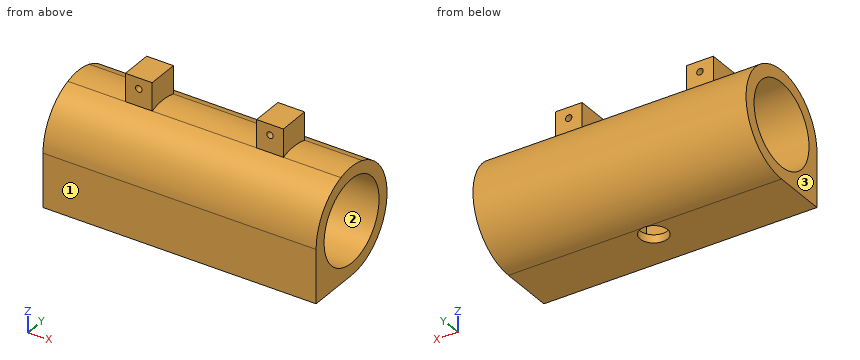
from build123d import *

# Parameters (mm, degrees)
SKETCH1_W                = 34
SKETCH1_H                = 30
BOSS_EXTRUDE2_DEPTH      = 51
SKETCH3_R                = 2.55
CUT_EXTRUDE3_DEPTH       = 10
SKETCH5_R                = 7.75
CUT_EXTRUDE4_DEPTH       = 51
SKETCH6_W                = 7
SKETCH6_H                = 30
CUT_EXTRUDE6_DEPTH       = 51
CUT_EXTRUDE7_DEPTH       = 51
CUT_EXTRUDE9_DEPTH       = 1.5
CUT_EXTRUDE9_DEPTH_BACK  = 1.5
BOSS_EXTRUDE5_DEPTH      = 51
CUT_EXTRUDE10_DEPTH      = 13
CUT_EXTRUDE11_DEPTH      = 13
SKETCH13_W               = 2
SKETCH13_H               = 6
CUT_EXTRUDE12_DEPTH      = 2
CUT_EXTRUDE13_DEPTH      = 13
CUT_EXTRUDE13_DEPTH_BACK = 11
BOSS_EXTRUDE6_DEPTH      = 2.25
BOSS_EXTRUDE7_DEPTH      = 2.25
BOSS_EXTRUDE8_DEPTH      = 2.25
BOSS_EXTRUDE9_DEPTH      = 2.25
SKETCH22_W               = 5
SKETCH22_H               = 6
BOSS_EXTRUDE10_DEPTH     = 1
SKETCH24_W               = 5
SKETCH24_H               = 6
BOSS_EXTRUDE11_DEPTH     = 1
SKETCH25_R               = 0.6
CUT_EXTRUDE14_DEPTH      = 20


with BuildPart() as part:
    # Sketch1 → Boss-Extrude2 (new body)
    with BuildSketch(Plane(origin=(0, 0, 0), x_dir=(0, 0, -1), z_dir=(1, 0, 0))):
        with Locations((-3.945183, 6.145902)):
            Rectangle(SKETCH1_W, SKETCH1_H)
    extrude(amount=BOSS_EXTRUDE2_DEPTH)

    # Sketch3 → Cut-Extrude3 (cut)
    with BuildSketch(Plane(origin=(0, 0, -13.054817), x_dir=(-1, 0, 0), z_dir=(0, 0, -1))):
        with Locations((-25.5, -1.354098)):
            Circle(SKETCH3_R)
    extrude(amount=-CUT_EXTRUDE3_DEPTH, mode=Mode.SUBTRACT)

    # Sketch5 → Cut-Extrude4 (cut)
    with BuildSketch(Plane(origin=(51, 0, 0), x_dir=(0, 0, -1), z_dir=(1, 0, 0))):
        with Locations((-3.945183, 1.145902)):
            Circle(SKETCH5_R)
    extrude(amount=-CUT_EXTRUDE4_DEPTH, mode=Mode.SUBTRACT)

    # Sketch6 → Cut-Extrude6 (cut)
    with BuildSketch(Plane(origin=(51, 0, 0), x_dir=(0, 0, -1), z_dir=(1, 0, 0))):
        with Locations((9.554817, 6.145902)):
            Rectangle(SKETCH6_W, SKETCH6_H)
    extrude(amount=-CUT_EXTRUDE6_DEPTH, mode=Mode.SUBTRACT)

    # Sketch7 → Cut-Extrude7 (cut)
    with BuildSketch(Plane(origin=(51, 0, 0), x_dir=(0, 0, -1), z_dir=(1, 0, 0))):
        with BuildLine():
            Line((-3.945183, -8.854098), (-20.945183, -8.854098))
            Line((-20.945183, -8.854098), (-20.945183, 21.145902))
            Line((-20.945183, 21.145902), (6.054817, 21.145902))
            Line((6.054817, 21.145902), (6.054817, 1.145902))
            ThreePointArc((6.054817, 1.145902), (-11.016251, 8.21697), (-3.945183, -8.854098))
        make_face()
    extrude(amount=-CUT_EXTRUDE7_DEPTH, mode=Mode.SUBTRACT)

    # Sketch8 → Cut-Extrude9 (cut, two sides)
    with BuildSketch(Plane(origin=(0, 0, -3.054817), x_dir=(-1, 0, 0), z_dir=(0, 0, -1))) as cut_extrude9_sk:
        Polygon((-21.75, -2.180132), (-21.75, -4.904098), (-29.25, -4.904098), (-29.25, -2.180132), (-29.25, 2.195902), (-21.75, 2.195902), align=None)
    extrude(amount=CUT_EXTRUDE9_DEPTH, mode=Mode.SUBTRACT)
    extrude(cut_extrude9_sk.sketch, amount=-CUT_EXTRUDE9_DEPTH_BACK, mode=Mode.SUBTRACT)

    # Sketch10 → Boss-Extrude5 (add)
    with BuildSketch(Plane(origin=(51, 0, 0), x_dir=(0, 0, -1), z_dir=(1, 0, 0))):
        Polygon((-17.695183, 1.145902), (-17.695183, 4.145902), (-11.695183, 4.145902), (-11.695183, 1.145902), (-11.695183, -1.854098), (-17.695183, -1.854098), align=None)
    extrude(amount=-BOSS_EXTRUDE5_DEPTH)

    # Sketch11 → Cut-Extrude10 (cut)
    with BuildSketch(Plane(origin=(51, 0, 0), x_dir=(0, 0, -1), z_dir=(1, 0, 0))):
        with BuildLine():
            Line((-13.484575, -1.854098), (-17.695183, -1.854098))
            Line((-17.695183, -1.854098), (-17.695183, 4.145902))
            Line((-17.695183, 4.145902), (-13.484575, 4.145902))
            ThreePointArc((-13.484575, 4.145902), (-13.945183, 1.145902), (-13.484575, -1.854098))
        make_face()
    extrude(amount=-CUT_EXTRUDE10_DEPTH, mode=Mode.SUBTRACT)

    # Sketch12 → Cut-Extrude11 (cut)
    with BuildSketch(Plane.ZY):
        with BuildLine():
            Line((13.484575, -1.854098), (17.695183, -1.854098))
            Line((17.695183, -1.854098), (17.695183, 4.145902))
            Line((17.695183, 4.145902), (13.484575, 4.145902))
            ThreePointArc((13.484575, 4.145902), (13.945183, 1.145902), (13.484575, -1.854098))
        make_face()
    extrude(amount=-CUT_EXTRUDE11_DEPTH, mode=Mode.SUBTRACT)

    # Sketch13 → Cut-Extrude12 (cut)
    with BuildSketch(Plane.XY.offset(17.695183)):
        with Locations((25.5, 1.145902)):
            Rectangle(SKETCH13_W, SKETCH13_H)
    extrude(amount=-CUT_EXTRUDE12_DEPTH, mode=Mode.SUBTRACT)

    # Sketch15 → Cut-Extrude13 (cut, two sides)
    with BuildSketch(Plane(origin=(24.5, 0, 0), x_dir=(0, 0, -1), z_dir=(1, 0, 0))) as cut_extrude13_sk:
        with BuildLine():
            Line((-17.695183, 4.145902), (-17.695183, -1.854098))
            Line((-17.695183, -1.854098), (-13.484575, -1.854098))
            ThreePointArc((-13.484575, -1.854098), (-13.945183, 1.145902), (-13.484575, 4.145902))
            Line((-13.484575, 4.145902), (-17.695183, 4.145902))
        make_face()
    extrude(amount=CUT_EXTRUDE13_DEPTH, mode=Mode.SUBTRACT)
    extrude(cut_extrude13_sk.sketch, amount=-CUT_EXTRUDE13_DEPTH_BACK, mode=Mode.SUBTRACT)

    # Sketch17 → Boss-Extrude6 (add)
    with BuildSketch(Plane(origin=(38, 0, 0), x_dir=(0, 0, -1), z_dir=(1, 0, 0))):
        with BuildLine():
            Line((-13.484575, 4.145902), (-17.695183, 4.145902))
            Line((-17.695183, 4.145902), (-17.695183, -1.854098))
            Line((-17.695183, -1.854098), (-13.484575, -1.854098))
            ThreePointArc((-13.484575, -1.854098), (-13.945183, 1.145902), (-13.484575, 4.145902))
        make_face()
    extrude(amount=BOSS_EXTRUDE6_DEPTH)

    # Sketch19 → Boss-Extrude7 (add)
    with BuildSketch(Plane.ZY.offset(-13)):
        with BuildLine():
            Line((13.484575, 4.145902), (17.695183, 4.145902))
            Line((17.695183, 4.145902), (17.695183, -1.854098))
            Line((17.695183, -1.854098), (13.484575, -1.854098))
            ThreePointArc((13.484575, -1.854098), (13.945183, 1.145902), (13.484575, 4.145902))
        make_face()
    extrude(amount=BOSS_EXTRUDE7_DEPTH)

    # Sketch20 → Boss-Extrude8 (add)
    with BuildSketch(Plane(origin=(13.5, 0, 0), x_dir=(0, 0, -1), z_dir=(1, 0, 0))):
        with BuildLine():
            Line((-17.695183, -1.854098), (-17.695183, 4.145902))
            Line((-17.695183, 4.145902), (-13.484575, 4.145902))
            ThreePointArc((-13.484575, 4.145902), (-13.945183, 1.145902), (-13.484575, -1.854098))
            Line((-13.484575, -1.854098), (-17.695183, -1.854098))
        make_face()
    extrude(amount=BOSS_EXTRUDE8_DEPTH)

    # Sketch21 → Boss-Extrude9 (add)
    with BuildSketch(Plane.ZY.offset(-37.5)):
        with BuildLine():
            Line((13.484575, 4.145902), (17.695183, 4.145902))
            Line((17.695183, 4.145902), (17.695183, -1.854098))
            Line((17.695183, -1.854098), (13.484575, -1.854098))
            ThreePointArc((13.484575, -1.854098), (13.945183, 1.145902), (13.484575, 4.145902))
        make_face()
    extrude(amount=BOSS_EXTRUDE9_DEPTH)

    # Sketch22 → Boss-Extrude10 (add)
    with BuildSketch(Plane.XY.offset(17.695183)):
        with Locations((37.75, 1.145902)):
            Rectangle(SKETCH22_W, SKETCH22_H)
    extrude(amount=BOSS_EXTRUDE10_DEPTH)

    # Sketch24 → Boss-Extrude11 (add)
    with BuildSketch(Plane.XY.offset(17.695183)):
        with Locations((13.25, 1.145902)):
            Rectangle(SKETCH24_W, SKETCH24_H)
    extrude(amount=BOSS_EXTRUDE11_DEPTH)

    # Sketch25 → Cut-Extrude14 (cut)
    with BuildSketch(Plane(origin=(0, 4.145902, 0), x_dir=(1, 0, 0), z_dir=(0, 1, 0))):
        with Locations((13.25, -16.695183)):
            Circle(SKETCH25_R)
        with Locations((37.75, -16.695183)):
            Circle(SKETCH25_R)
    extrude(amount=-CUT_EXTRUDE14_DEPTH, mode=Mode.SUBTRACT)


solid = part.part
Verification items for the finished model (mm, model axes). Face numbers are marked on the shaded views. Give positions to 0.01 mm unless a question says otherwise; leave off trailing zeros. Loops run counter-clockwise (first coordinate to the right, second up) from the corner with the lowest first, then second, coordinate; pieces in that order, holes last.
1) Sectioned sample at D-D, the plane y = -3. Enter the section's corners in (x, z).
2) Thickness scan on line 1 along Y through (x, z) = (3, 4.25); line 2 along Z through (x, y) = (43, 1.5); line 3 along X through (y, z) = (-1, 15.25). Record the ranges inside material, lowest first.
3) Sectioned sample at C-C, the plane z = 2.5. Enter the section's corners in (x, y).
4) Draft check along Y on the marked faces 1, 2 and 3. Enter one of: pulls with the +Y half, pulls with the -Y half, needs draft (parallel to the pull), parting line crosses it, or undercut.
5) Depth check by flat-ended pin: pin 1 Ø2 at (x, y) = (25, -2.5) entering from +Z; pin 2 Ø1.6 at (x, z) = (37.75, 16.7) entering from +Y; pin 3 Ø4 at (y, z) = (2.5, 16) entering from -X. Enter the tip coordinate at first touch or a pass-through.
6) Sectioned sample at B-B, the plane x = 48. Enter the section's corners in (y, z), then the cut area to 3 significant figures.
7) Sectioned sample at A-A, the plane x = 37.75. Enter the section's corners in (y, z).
Answers:
1. outline: (0, -6.05) - (23.55, -6.05) - (23.55, -4.55) - (21.75, -4.55) - (21.75, -2.6) - (0, -2.6) - close; (0, 10.49) - (51, 10.49) - (51, 13.05) - (0, 13.05) - close; (27.45, -6.05) - (51, -6.05) - (51, -2.6) - (29.25, -2.6) - (29.25, -4.55) - (27.45, -4.55) - close
2. line 1: y = -8.85 to -6.6, 8.89 to 11.14
2. line 2: z = -6.05 to -3.8, 11.69 to 13.94
2. line 3: x = 10.75 to 15.75, 35.25 to 40.25
3. outline: (0, -8.85) - (51, -8.85) - (51, -6.47) - (0, -6.47) - close; (0, 8.76) - (51, 8.76) - (51, 11.04) - (0, 11.04) - close
4. face 1: pulls with the -Y half
4. face 2: undercut
4. face 3: needs draft
5. pin 1: stops at z = 13.59
5. pin 2: stops at y = 4.15
5. pin 3: stops at x = 10.75
6. outline: (-8.85, -6.05) - (1.15, -6.05) arc R10 ccw (long way) to (-8.85, 3.95) - close; hole circle Ø15.5 at (1.15, 3.95)
6. area: 147 mm2
7. outline: (-8.85, -6.05) - (1.15, -6.05) arc R10 ccw to (4.15, 13.48) - (4.15, 16.1) - (-1.85, 16.1) - (-1.85, 13.48) arc R10 ccw to (-8.85, 3.95) - close; (-1.85, 17.3) - (4.15, 17.3) - (4.15, 18.7) - (-1.85, 18.7) - close; hole circle Ø15.5 at (1.15, 3.95)
